```python
from build123d import *

# Parameters (mm, degrees)
BOSS_EXTRUDE1_DEPTH = 3
SKETCH2_R           = 1
SKETCH2_W           = 9
SKETCH2_H           = 9
CUT_EXTRUDE1_DEPTH  = 3


with BuildPart() as part:
    # Sketch1 → Boss-Extrude1 (new body)
    with BuildSketch(Plane.XY):
        Polygon((-35, 38), (-17.5, 38), (17.5, 38), (35, 38), (35, 20.5), (38, 20.5), (38, -20.5), (35, -20.5), (35, -38), (35, -41), (17.5, -41), (17.5, -38), (-17.5, -38), (-17.5, -41), (-35, -41), (-38, -41), (-38, -38), (-38, -20.5), (-35, -20.5), (-35, 20.5), (-38, 20.5), (-38, 38), align=None)
    extrude(amount=BOSS_EXTRUDE1_DEPTH)

    # Sketch2 → Cut-Extrude1 (cut)
    with BuildSketch(Plane.XY.offset(3)):
        with Locations((-10.5, 12.5)):
            Circle(SKETCH2_R)
        with Locations((-10.5, 0)):
            Circle(SKETCH2_R)
        with Locations((10.5, 12.5)):
            Circle(SKETCH2_R)
        with Locations((10.5, 0)):
            Circle(SKETCH2_R)
        Rectangle(SKETCH2_W, SKETCH2_H)
    extrude(amount=-CUT_EXTRUDE1_DEPTH, mode=Mode.SUBTRACT)


solid = part.part
```
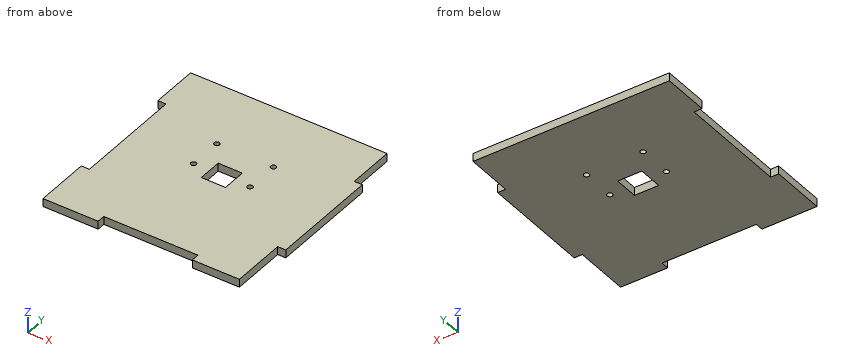
Could you check a few things on this model? Use its own coordinates, in mm. Give positions to 0.01 mm unless a question says otherwise; leave off trailing zeros. Loops run counter-clockwise (first coordinate to the right, second up) from the corner with the lowest first, then second, coordinate; pieces in that order, holes last. Notation, with made-up numbers: (-25, 22.25) - (30, 22.25) arc R24 cw to (30, 51.25) - close; hole circle Ø3 at (22.25, 26.5). An arc over 180 degrees is marked (long way). Answer in a Markdown table with one row per item. Add a question column.
Q1. Please list where these lines run through material, in increasing order: L1, parallel to Y at x = -10.5, z = 1.7; L2, parallel to Y at x = -4, z = 0.75; L3, parallel to Y at x = -12, z = 0.3. Write a range as from..to.
Q2. If we section it at A-A (x = -0.5): List the corners of the cut face in (y, z) for me, plus the area to 3 significant figures.
Q3. For pin 1 (1.2 mm diameter, centred on x = 10.5, y = 12.5, fed in from +Z); pin 2 (0.9 mm diameter, centred on x = 36, z = 2, fed in from -Y); pin 3 (0.9 mm diameter, centred on y = -35.5, z = 1, fed in from +X), each with a flat end and sliding along its axis, tell me the tip position at first contact or that it passes through.
Q4. If we section it at C-C (z = 1.35): List the corners of the cut face in (x, y) for me.
Q5. If we section it at D-D (y = 12.5): List the corners of the cut face in (x, z) for me, plus the area to 3 significant figures.
Q6. If we section it at B-B (y = 0): List the corners of the cut face in (x, z) for me.
The answers:
| question | item | result |
|---|---|---|
| 1 | L1 | y = -38..-1, 1..11.5, 13.5..38 |
| 1 | L2 | y = -38..-4.5, 4.5..38 |
| 1 | L3 | y = -38..38 |
| 2 | outline | (-38, 0) - (-4.5, 0) - (-4.5, 3) - (-38, 3) - close; (4.5, 0) - (38, 0) - (38, 3) - (4.5, 3) - close |
| 2 | area | 201 mm^2 |
| 3 | pin 1 | passes through |
| 3 | pin 2 | stops at y = -20.5 |
| 3 | pin 3 | stops at x = 35 |
| 4 | outline | (-38, -41) - (-17.5, -41) - (-17.5, -38) - (17.5, -38) - (17.5, -41) - (35, -41) - (35, -20.5) - (38, -20.5) - (38, 20.5) - (35, 20.5) - (35, 38) - (-38, 38) - (-38, 20.5) - (-35, 20.5) - (-35, -20.5) - (-38, -20.5) - close; hole circle Ø2 at (-10.5, 0); hole circle Ø2 at (-10.5, 12.5); hole (-4.5, -4.5) - (4.5, -4.5) - (4.5, 4.5) - (-4.5, 4.5) - close; hole circle Ø2 at (10.5, 0); hole circle Ø2 at (10.5, 12.5) |
| 5 | outline | (-35, 0) - (-11.5, 0) - (-11.5, 3) - (-35, 3) - close; (-9.5, 0) - (9.5, 0) - (9.5, 3) - (-9.5, 3) - close; (11.5, 0) - (38, 0) - (38, 3) - (11.5, 3) - close |
| 5 | area | 207 mm^2 |
| 6 | outline | (-35, 0) - (-11.5, 0) - (-11.5, 3) - (-35, 3) - close; (-9.5, 0) - (-4.5, 0) - (-4.5, 3) - (-9.5, 3) - close; (4.5, 0) - (9.5, 0) - (9.5, 3) - (4.5, 3) - close; (11.5, 0) - (38, 0) - (38, 3) - (11.5, 3) - close |
